Input: part model. Units: mm. Frame: model coordinates. A direction names the side the tool comes from. Round coordinates to 2 decimals unless told otherwise and drop trailing zeros. Loops run counter-clockwise (first coordinate to the right, second up) from the corner with the lowest first, then second, coordinate; pieces in that order, holes last.
1) Section A-A, the plane x = -50. Return loops of the section in (y, z).
2) Ray query, line 1 along X through (y, z) = (-4, 2.05); line 2 along Y through (x, z) = (17.5, 1.4); line 3 along Y through (x, z) = (-42, 0.85). Return the intervals inside material, ascending.
3) First-contact query: pin 1 (3.5 mm diameter, centred on x = 10, y = 0, fed in from +Z); pin 2 (1.5 mm diameter, centred on y = 119.5, z = 2.5, fed in from -X); pin 3 (1.5 mm diameter, centred on x = 41, z = 1, fed in from +Y); pin 4 (1.5 mm diameter, centred on y = 7, z = 1, fed in from -X). Flat tips, straight axial feed; report the tip coordinate or a pass-through.
4) Section D-D, the plane y = -33.5. Return loops of the section in (x, z).
5) Section C-C, the plane z = 2.35. State how many separate pieces and enclosed holes the cut face has, and give its area (3 significant figures).
6) Access query for faces 5 (the face through (106.937, 147.861, 1.479)), 6 (the face through (66.46, -115.17, 1.48)), 7 (the face through (-2, 2, 3)), 8 (the face through (98, 157.06, 1.48)), 9 (the face through (-107.06, 148, 1.48)). Directions: +Z, -Z, +X, -X, +Y, -Y. A direction counts if a zero-diameter tool reaches every point of the face in a straight line with its end or side. Return the directions, or none.
7) Draft query along Y for faces 1 (the face through (-97.861, 156.937, 1.479)), 2 (the face through (-66.46, 115.17, 1.48)), 3 (the face through (47.6, -16.3, 1.5)), 4 (the face through (-2, 2, 0)). Return one class per face: pulls with the +Y half, pulls with the -Y half, needs draft (parallel to the pull), parting line crosses it, or undercut.
8) Section B-B, the plane y = 66. Return loops of the section in (x, z) (3 decimals), and give its area (3 significant figures).
from build123d import *

# Parameters (mm, degrees)
MODEL_R                 = 1.55
MODEL_R_2               = 2.05
SALIENTE_EXTRUIR1_DEPTH = 3


with BuildPart() as part:
    # Model → Saliente-Extruir1 (new body)
    with BuildSketch(Plane.XY):
        with BuildLine():
            Line((-102.502115315, -142.835304077), (-111.498730811, -153.029934372))
            ThreePointArc((-111.498730811, -153.029934372), (-112.469021565, -159.467752645), (-107, -163))
            Line((-107, -163), (-0.700702433, -163))
            Line((-0.700702433, -163), (0, -160.996661892))
            Line((0, -160.996661892), (0.699463472, -163))
            Line((0.699463472, -163), (107, -163))
            ThreePointArc((107, -163), (112.469021565, -159.467752645), (111.498730811, -153.029934372))
            Line((111.498730811, -153.029934372), (102.502115315, -142.835304077))
            ThreePointArc((102.502115315, -142.835304077), (100.646421892, -139.755557374), (100, -136.21852803))
            Line((100, -136.21852803), (100, -107))
            Line((100, -107), (105, -102))
            Line((105, -102), (105, 102))
            Line((105, 102), (100, 107))
            Line((100, 107), (100, 136.21852803))
            ThreePointArc((100, 136.21852803), (100.646421892, 139.755557374), (102.502115315, 142.835304077))
            Line((102.502115315, 142.835304077), (111.498730811, 153.029934372))
            ThreePointArc((111.498730811, 153.029934372), (111.242640687, 161.242640687), (103.029934372, 161.498730811))
            Line((103.029934372, 161.498730811), (92.835304077, 152.502115315))
            ThreePointArc((92.835304077, 152.502115315), (89.755557374, 150.646421892), (86.21852803, 150))
            Line((86.21852803, 150), (0.701283747, 150))
            Line((0.701283747, 150), (0, 148))
            Line((0, 148), (-0.697387345, 150))
            Line((-0.697387345, 150), (-86.21852803, 150))
            ThreePointArc((-86.21852803, 150), (-89.755557374, 150.646421892), (-92.835304077, 152.502115315))
            Line((-92.835304077, 152.502115315), (-103.029934372, 161.498730811))
            ThreePointArc((-103.029934372, 161.498730811), (-111.242640687, 161.242640687), (-111.498730811, 153.029934372))
            Line((-111.498730811, 153.029934372), (-102.502115315, 142.835304077))
            ThreePointArc((-102.502115315, 142.835304077), (-100.646421892, 139.755557374), (-100, 136.21852803))
            Line((-100, 136.21852803), (-100, 107))
            Line((-100, 107), (-105, 102))
            Line((-105, 102), (-105, -102))
            Line((-105, -102), (-100, -107))
            Line((-100, -107), (-100, -136.21852803))
            ThreePointArc((-100, -136.21852803), (-100.646421892, -139.755557374), (-102.502115315, -142.835304077))
        make_face()
        with Locations((-104.5, -154)):
            Circle(MODEL_R, mode=Mode.SUBTRACT)
        with Locations((104.5, -154)):
            Circle(MODEL_R, mode=Mode.SUBTRACT)
        with Locations((-10, 0)):
            Circle(MODEL_R_2, mode=Mode.SUBTRACT)
        with Locations((0, -15)):
            Circle(MODEL_R_2, mode=Mode.SUBTRACT)
        with Locations((10, 0)):
            Circle(MODEL_R_2, mode=Mode.SUBTRACT)
        with Locations((0, 15)):
            Circle(MODEL_R_2, mode=Mode.SUBTRACT)
        with Locations((104.5, 155)):
            Circle(MODEL_R, mode=Mode.SUBTRACT)
        with Locations((-104.5, 155)):
            Circle(MODEL_R, mode=Mode.SUBTRACT)
        with BuildLine():
            Line((24.151525156, -40), (-24.151525156, -40))
            ThreePointArc((-24.151525156, -40), (-29.19998413, -41.367905122), (-32.867280527, -45.097387604))
            Line((-32.867280527, -45.097387604), (-66.617280527, -105.097387604))
            ThreePointArc((-66.617280527, -105.097387604), (-66.533620034, -115.048458975), (-57.901525156, -120))
            Line((-57.901525156, -120), (57.901525156, -120))
            ThreePointArc((57.901525156, -120), (66.533620034, -115.048458975), (66.617280527, -105.097387604))
            Line((66.617280527, -105.097387604), (32.867280527, -45.097387604))
            ThreePointArc((32.867280527, -45.097387604), (29.19998413, -41.367905122), (24.151525156, -40))
        make_face(mode=Mode.SUBTRACT)
        with BuildLine():
            Line((32.867280527, 45.097387604), (66.617280527, 105.097387604))
            ThreePointArc((66.617280527, 105.097387604), (66.533620034, 115.048458975), (57.901525156, 120))
            Line((57.901525156, 120), (-57.901525156, 120))
            ThreePointArc((-57.901525156, 120), (-66.533620034, 115.048458975), (-66.617280527, 105.097387604))
            Line((-66.617280527, 105.097387604), (-32.867280527, 45.097387604))
            ThreePointArc((-32.867280527, 45.097387604), (-29.19998413, 41.367905122), (-24.151525156, 40))
            Line((-24.151525156, 40), (24.151525156, 40))
            ThreePointArc((24.151525156, 40), (29.19998413, 41.367905122), (32.867280527, 45.097387604))
        make_face(mode=Mode.SUBTRACT)
        with BuildLine():
            Line((-37.763932023, 11.381966011), (-57.763932023, 21.381966011))
            ThreePointArc((-57.763932023, 21.381966011), (-62.628655561, 21.163084098), (-65, 16.909830056))
            Line((-65, 16.909830056), (-65, -16.909830056))
            ThreePointArc((-65, -16.909830056), (-62.628655561, -21.163084098), (-57.763932023, -21.381966011))
            Line((-57.763932023, -21.381966011), (-37.763932023, -11.381966011))
            ThreePointArc((-37.763932023, -11.381966011), (-35.746745958, -9.538485617), (-35, -6.909830056))
            Line((-35, -6.909830056), (-35, 6.909830056))
            ThreePointArc((-35, 6.909830056), (-35.746745958, 9.538485617), (-37.763932023, 11.381966011))
        make_face(mode=Mode.SUBTRACT)
        with BuildLine():
            Line((37.763932023, -11.381966011), (57.763932023, -21.381966011))
            ThreePointArc((57.763932023, -21.381966011), (62.628655561, -21.163084098), (65, -16.909830056))
            Line((65, -16.909830056), (65, 16.909830056))
            ThreePointArc((65, 16.909830056), (62.628655561, 21.163084098), (57.763932023, 21.381966011))
            Line((57.763932023, 21.381966011), (37.763932023, 11.381966011))
            ThreePointArc((37.763932023, 11.381966011), (35.746745958, 9.538485617), (35, 6.909830056))
            Line((35, 6.909830056), (35, -6.909830056))
            ThreePointArc((35, -6.909830056), (35.746745958, -9.538485617), (37.763932023, -11.381966011))
        make_face(mode=Mode.SUBTRACT)
    extrude(amount=SALIENTE_EXTRUIR1_DEPTH)


solid = part.part
Final values:
1. outline: (-163, 0) - (-120, 0) - (-120, 3) - (-163, 3) - close; (-75.56, 0) - (-17.5, 0) - (-17.5, 3) - (-75.56, 3) - close; (17.5, 0) - (75.56, 0) - (75.56, 3) - (17.5, 3) - close; (120, 0) - (150, 0) - (150, 3) - (120, 3) - close
2. line 1: x = -105 to -65, -35 to 35, 65 to 105
2. line 2: y = -163 to -120, -40 to 40, 120 to 150
2. line 3: y = -163 to -120, -61.33 to -13.5, 13.5 to 61.33, 120 to 150
3. pin 1: passes through
3. pin 2: stops at x = -100
3. pin 3: stops at y = 150
3. pin 4: stops at x = -105
4. outline: (-105, 0) - (105, 0) - (105, 3) - (-105, 3) - close
5. separate pieces: 1
5. enclosed holes: 12
5. area: 46,900 mm2
6. face 5: +Z, -Z, +X
6. face 6: +Z, -Z
6. face 7: +Z, +X, -X, +Y, -Y
6. face 8: +Z, -Z, +Y
6. face 9: +Z, -Z, -X
7. face 1: pulls with the +Y half
7. face 2: undercut
7. face 3: undercut
7. face 4: needs draft
8. outline: (-105, 0) - (-44.625, 0) - (-44.625, 3) - (-105, 3) - close; (44.625, 0) - (105, 0) - (105, 3) - (44.625, 3) - close
8. area: 362 mm2
